```python
from build123d import *

# Parameters (mm, degrees)
SKETCH1_R           = 15
BOSS_EXTRUDE1_DEPTH = 6
CUT_EXTRUDE1_DEPTH  = 6


with BuildPart() as part:
    # Sketch1 → Boss-Extrude1 (new body)
    with BuildSketch(Plane(origin=(0, 0, 0), x_dir=(1, 0, 0), z_dir=(0, 1, 0))):
        with BuildLine():
            Line((-7.12002198, 13.202472761), (-11.849818066, 19.712478581))
            Line((-11.849818066, 19.712478581), (-15.085886044, 17.361337572))
            Line((-15.085886044, 17.361337572), (-10.356089958, 10.851331752))
            ThreePointArc((-10.356089958, 10.851331752), (-8.816778784, 12.135254916), (-7.12002198, 13.202472761))
        make_face()
        with BuildLine():
            Line((2, 22.912878475), (-2, 22.912878475))
            Line((-2, 22.912878475), (-2, 14.866068747))
            ThreePointArc((-2, 14.866068747), (0, 15), (2, 14.866068747))
            Line((2, 14.866068747), (2, 22.912878475))
        make_face()
        with BuildLine():
            Line((15.085886044, 17.361337572), (11.849818066, 19.712478581))
            Line((11.849818066, 19.712478581), (7.12002198, 13.202472761))
            ThreePointArc((7.12002198, 13.202472761), (8.816778784, 12.135254916), (10.356089958, 10.851331752))
            Line((10.356089958, 10.851331752), (15.085886044, 17.361337572))
        make_face()
        with BuildLine():
            Line((22.409476369, 5.178355806), (21.173408392, 8.982581871))
            Line((21.173408392, 8.982581871), (13.520437565, 6.495980915))
            ThreePointArc((13.520437565, 6.495980915), (14.265847744, 4.635254916), (14.756505543, 2.69175485))
            Line((14.756505543, 2.69175485), (22.409476369, 5.178355806))
        make_face()
        Circle(SKETCH1_R)
        with BuildLine():
            Line((21.173408392, -8.982581871), (22.409476369, -5.178355806))
            Line((22.409476369, -5.178355806), (14.756505543, -2.69175485))
            ThreePointArc((14.756505543, -2.69175485), (14.265847744, -4.635254916), (13.520437565, -6.495980915))
            Line((13.520437565, -6.495980915), (21.173408392, -8.982581871))
        make_face()
        with BuildLine():
            Line((11.849818066, -19.712478581), (15.085886044, -17.361337572))
            Line((15.085886044, -17.361337572), (10.356089958, -10.851331752))
            ThreePointArc((10.356089958, -10.851331752), (8.816778784, -12.135254916), (7.12002198, -13.202472761))
            Line((7.12002198, -13.202472761), (11.849818066, -19.712478581))
        make_face()
        with BuildLine():
            Line((-2, -14.866068747), (-2, -22.912878475))
            Line((-2, -22.912878475), (2, -22.912878475))
            Line((2, -22.912878475), (2, -14.866068747))
            ThreePointArc((2, -14.866068747), (0, -15), (-2, -14.866068747))
        make_face()
        with BuildLine():
            Line((-10.356089958, -10.851331752), (-15.085886044, -17.361337572))
            Line((-15.085886044, -17.361337572), (-11.849818066, -19.712478581))
            Line((-11.849818066, -19.712478581), (-7.12002198, -13.202472761))
            ThreePointArc((-7.12002198, -13.202472761), (-8.816778784, -12.135254916), (-10.356089958, -10.851331752))
        make_face()
        with BuildLine():
            Line((-14.756505543, -2.69175485), (-22.409476369, -5.178355806))
            Line((-22.409476369, -5.178355806), (-21.173408392, -8.982581871))
            Line((-21.173408392, -8.982581871), (-13.520437565, -6.495980915))
            ThreePointArc((-13.520437565, -6.495980915), (-14.265847744, -4.635254916), (-14.756505543, -2.69175485))
        make_face()
        with BuildLine():
            Line((-13.520437565, 6.495980915), (-21.173408392, 8.982581871))
            Line((-21.173408392, 8.982581871), (-22.409476369, 5.178355806))
            Line((-22.409476369, 5.178355806), (-14.756505543, 2.69175485))
            ThreePointArc((-14.756505543, 2.69175485), (-14.265847744, 4.635254916), (-13.520437565, 6.495980915))
        make_face()
    extrude(amount=BOSS_EXTRUDE1_DEPTH)

    # Sketch2 → Cut-Extrude1 (cut)
    with BuildSketch(Plane(origin=(0, 6, 0), x_dir=(1, 0, 0), z_dir=(0, 1, 0))):
        with BuildLine():
            Line((1.401998573, 2.13), (-1.401998573, 2.13))
            ThreePointArc((-1.401998573, 2.13), (-1.209835451, -2.24472675), (2.55, 0))
            ThreePointArc((2.55, 0), (2.24472675, 1.209835451), (1.401998573, 2.13))
        make_face()
    extrude(amount=-CUT_EXTRUDE1_DEPTH, mode=Mode.SUBTRACT)


solid = part.part
```
Here's how the part is built. I have some questions about the finished solid (model axes, mm). A direction names the side the tool comes from. Coordinates: 2 decimals unless noted, no trailing zeros. Loops run counter-clockwise (first coordinate to the right, second up) from the corner with the lowest first, then second, coordinate; pieces in that order, holes last. Notation, with made-up numbers: (-24, 9) -> (21, 9) arc R21 cw to (21, 18) -> close; hole circle Ø8 at (27.5, 45.5). An arc over 180 degrees is marked (long way). Return JSON: item names as keys, results as strings.
1) For faces 1 (the face through (12.688, 2.958, -14.061)), 2 (the face through (2, 3, 19)), 3 (the face through (-2, 3, -19)), which set-ups out of +Z, -Z, +X, -X, +Y, -Y let a thin tool reach every point of the face, with its end or its side?
Results below:
{"face 1": "+X, +Y, -Y", "face 2": "+Z, +Y, -Y", "face 3": "-Z, +Y, -Y"}
2) Will these pins go through, and if not, where does the flat tip stop? pin 1 (1.8 mm diameter, centred on y = 3, z = 18.5, fed in from -X); pin 2 (1 mm diameter, centred on x = 16.5, y = 4.5, fed in from -Z); pin 3 (3 mm diameter, centred on y = 3.5, z = -17, fed in from -X).
Results below:
{"pin 1": "x = -14.76", "pin 2": "z = -7.63", "pin 3": "x = -15.09"}
3) If we section it at B-B, the plane x = 6.5: Write out the boundary of the cut face in (y, z).
Results below:
{"outline": "(0, -13.52) -> (6, -13.52) -> (6, 13.52) -> (0, 13.52) -> close"}
4) If we section it at A-A, the plane x = 0: Write out the boundary of the cut face in (y, z), then the cut area to 3 significant figures.
Results below:
{"outline": "(0, -22.91) -> (6, -22.91) -> (6, -2.13) -> (0, -2.13) -> close; (0, 2.55) -> (6, 2.55) -> (6, 22.91) -> (0, 22.91) -> close", "area": "247 mm²"}
5) If we section it at C-C, the plane x = -9: Write out the boundary of the cut face in (y, z).
Results below:
{"outline": "(0, -15.79) -> (6, -15.79) -> (6, 15.79) -> (0, 15.79) -> close"}
6) I need wall thicknesses on line 1 (Z direction, x = 0, y = 3.5); line 2 (Z direction, x = 11.5, y = 0.55); line 3 (X direction, y = 1.5, z = -18). Which ranges of each line are inside material? Lowest first, please. Write a range as from..to.
Results below:
{"line 1": "-22.91..-2.13, 2.55..22.91", "line 2": "-19.23..-12.43, -9.63..9.63, 12.43..19.23", "line 3": "-14.21..-10.61, -2..2, 10.61..14.21"}
7) Thinking about a two-plate mould opening in X: for faces 4 (the face through (9.518, 2.958, -16.503)), 5 (the face through (-12.688, 2.958, 14.061)), 6 (the face through (13.45, 2.96, 18.55)), which applies, +X half, -X half, draft (parallel to the pull), parting line (faces both ways), or undercut?
Results below:
{"face 4": "undercut", "face 5": "-X half", "face 6": "+X half"}
